Autodesk Inventor part; units mm, degrees
ref_plane "Work Plane1" through (0, 0, 0) normal (0, 1, 0) x (0, 0, 1)
ref_plane "YZ Plane" through (0, 0, 0) normal (1, 0, 0) x (0, 1, 0)
ref_plane "XZ Plane" through (0, 0, 0) normal (0, 1, 0) x (-1, 0, 0)
sketch "Sketch1" plane through (0, 0, 0) normal (0, 0, 1) x (1, 0, 0)
  circle A0 centre (0, 0) radius 27.7812
  dimension "d0" = 55.5625
extrude "Extrusion1" add sketch "Sketch1" along normal blind 266.7
ref_plane "Work Plane1" through (0, 0, 0) normal (0, 1, 0) x (0, 0, 1)
sketch "Sketch2" plane through (0, 0, 0) normal (0, 1, 0) x (0, 0, 1)
  line L0 (-53.34, 0) -> (320.04, 0)
  line L1 (0, -24.6062) -> (60.325, -24.6062)
  line L2 (60.325, -24.6062) -> (63.5, -27.7812)
  line L3 (0, -27.7812) -> (266.7, -27.7812)
  line L4 (0, -24.6062) -> (0, -27.7812)
  line L5 (0, 27.7812) -> (0, -27.7812)
  dimension "d4" = 24.6062
  dimension "d5" = 135
  dimension "d6" = 60.325
revolve "Revolution1" cut sketch "Sketch2" angle 360 about axis through (0, 0, 0) along (0, 0, 1)
sketch "Sketch3" plane through (0, 0, 0) normal (0, 1, 0) x (0, 0, 1)
  line L0 (60.325, -24.6062) -> (0, -24.6062)
  line L1 (0, 24.6062) -> (0, -24.6062)
  line L2 (-127.1587, 0) -> (762.9525, 0)
  line L3 (0, -17.1768) -> (54.6612, -17.1767)
  arc A0 (85.725, -27.7812) -> (54.6612, -17.1767) centre (54.6612, -67.9767) ccw
  line L4 (60.325, 24.6062) -> (0, 24.6062)
  line L5 (63.5, -27.7812) -> (266.7, -27.7812)
  line L6 (63.5, -27.7812) -> (60.325, -24.6062)
  dimension "d8" = 50.8
  dimension "d9" = 41.783
  dimension "d10" = 85.725
extrude "Extrusion2" cut sketch "Sketch3" against normal mid plane 12.7
sketch "Sketch4" plane through (0, 0, 0) normal (0, 1, 0) x (0, 0, 1)
  line L0 (266.7, 27.7812) -> (266.7, -27.7812)
  line L1 (85.725, -27.7812) -> (266.7, -27.7812)
  line L2 (63.5, 27.7812) -> (266.7, 27.7812)
  line L3 (266.7, -20.4788) -> (165.1, -20.4788)
  arc A0 (165.1, -20.4788) -> (139.7, -27.7812) centre (165.1, -68.3039) ccw
  dimension "d13" = 101.6
  dimension "d14" = 127
  dimension "d15" = 48.26
extrude "Extrusion3" cut sketch "Sketch4" against normal mid plane 12.7
properties part number "shaft" material "Steel, Mild"
Design review of the part built by this model. Coordinates are the model's own, in mm. A direction names the side the tool comes from. Give positions to 0.01 mm unless a question says otherwise; leave off trailing zeros. Loops run counter-clockwise (first coordinate to the right, second up) from the corner with the lowest first, then second, coordinate; pieces in that order, holes last. Notation, with made-up numbers: (46.5, -18.75) -> (73.5, -18.75) arc R15 ccw to (73.5, 5.25) -> close; hole circle Ø10 at (-2, 18). An arc over 180 degrees is marked (long way). One line per item, written item: value.
Q1. Draft analysis for pull direction Y (two halves, no side actions). For faces 5 (the flat face through (-24, 6.35, 203)), 6 (the cylindrical face through (25.663, 10.64, 163.678)), 7 (the flat face through (0, 0, 266.7)), state which applies: pulls with the +Y half, pulls with the -Y half, needs draft (parallel to the pull), parting line crosses it, or undercut.
Numbers:
face 5: undercut
face 6: parting line crosses it
face 7: needs draft
Q2. We need section B-B on z = 170. Give the boundary of the cut face in (x, y).
Numbers:
outline: (-27.05, -6.35) arc R27.78 ccw (long way) to (-27.05, 6.35) -> (-20.48, 6.35) -> (-20.48, -6.35) -> close
Q3. We need section C-C on z = 47. Give the boundary of the cut face in (x, y), and give its area (3 significant figures).
Numbers:
outline: (-23.77, -6.35) arc R24.61 ccw (long way) to (-23.77, 6.35) -> (-17.18, 6.35) -> (-17.18, -6.35) -> close
area: 1,810 mm^2
Q4. For pin 1 Ø7 at (x, z) = (-23, 233) entering from -Y; pin 2 Ø5 at (x, z) = (-16, 234) entering from +Y; pin 3 Ø5 at (y, z) = (-13, 220) entering from +X; pin 4 Ø8 at (y, z) = (4, 227) entering from +X, all flat-tipped, find the tip position at first contact; note any pin that passes through.
Numbers:
pin 1: stops at y = -19.79
pin 2: stops at y = 24.28
pin 3: stops at x = 25.72
pin 4: stops at x = 27.78
Q5. We need section A-A on x = 0. Give the boundary of the cut face in (y, z) (3 decimals).
Numbers:
outline: (-27.781, 63.5) -> (-24.606, 60.325) -> (-24.606, 0) -> (24.606, 0) -> (24.606, 60.325) -> (27.781, 63.5) -> (27.781, 266.7) -> (-27.781, 266.7) -> close
Q6. For L1, parallel to Y at x = 1.5, z = 75; L2, parallel to Y at x = -0.5, z = 154; L3, parallel to X at y = 12, z = 122.5, list the stretches that pass through material, from the lowest coordinate up.
Numbers:
L1: y = -27.74 to 27.74
L2: y = -27.78 to 27.78
L3: x = -25.06 to 25.06
Q7. Machinability: for faces 1 (the flat face through (-24, -6.35, 203)), 2 (the cylindrical face through (24.586, -0.992, 30.585)), 3 (the flat face through (0, 0, 0)), 4 (the flat face through (-21, 6.35, 42)), which of the approach directions +Z, -Z, +X, -X, +Y, -Y give a long, thin tool a straight path to every point of the face, cutting with its end or side? Answer none if there is none.
Numbers:
face 1: +Z, -X
face 2: -Z
face 3: -Z, +X, -X, +Y, -Y
face 4: -Z, -X
